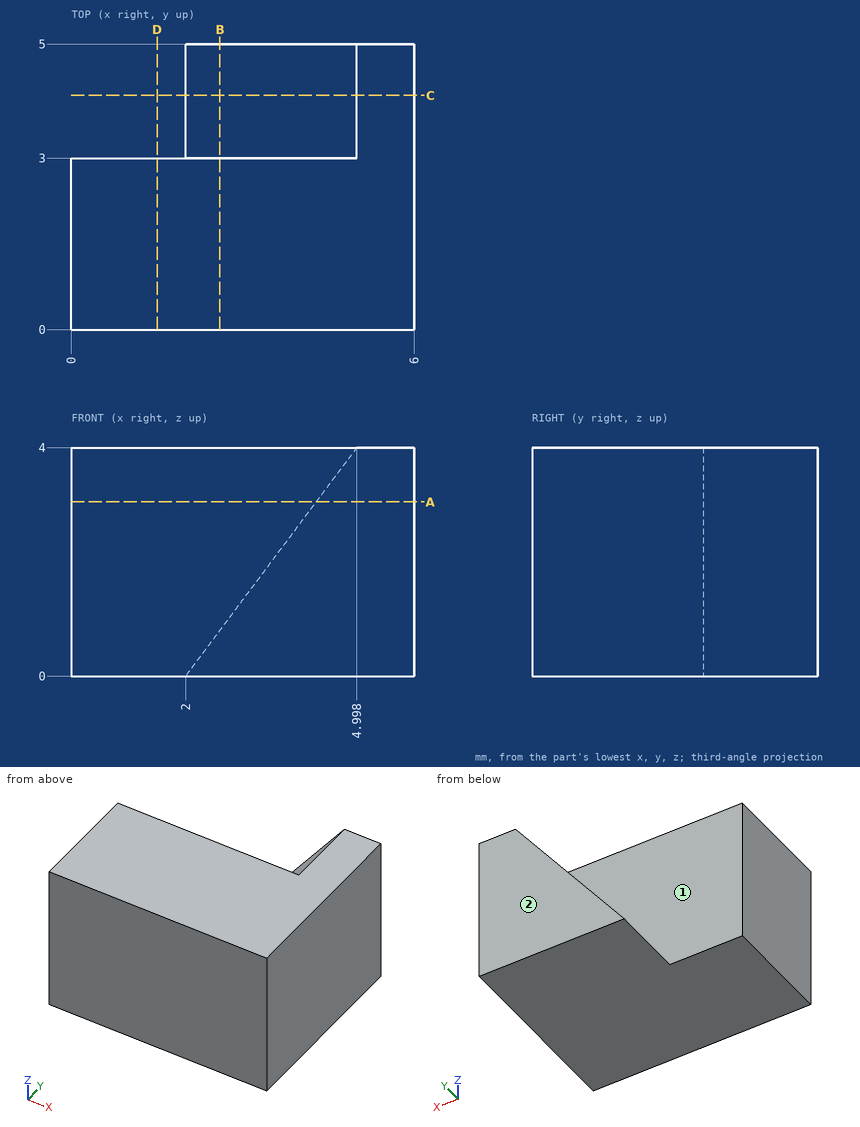
Part print with two shaded views. Sizes in mm from the minimum x, y, z corner. A direction names the side the tool comes from. Round coordinates to 2 decimals unless told otherwise and drop trailing zeros. Loops run counter-clockwise (first coordinate to the right, second up) from the corner with the lowest first, then second, coordinate; pieces in that order, holes last.
Item 1: Drill centre lines: line 1 along Y through (x, z) = (1.9, 1.45); line 2 along X through (y, z) = (4.45, 3.2); line 3 along X through (y, z) = (3.5, 1.85). Where is each one in solid material? Low to high.
Item 2: Which spindle directions (+Z, -Z, +X, -X, +Y, -Y) get a long thin tool onto all of the face, cutting with end or side? Do the marked faces 1 and 2. Say none if no direction does.
Item 3: Saw through at A-A (z = 3.05). List the corners of the cut face in (x, y), then the cut area to 3 significant figures.
Item 4: Saw through at D-D (x = 1.5). List the corners of the cut face in (y, z), then the cut area to 3 significant figures.
Item 5: Saw through at B-B (x = 2.6). List the corners of the cut face in (y, z), then the cut area to 3 significant figures.
Item 6: Saw through at C-C (y = 4.1). List the corners of the cut face in (x, z), then the cut area to 3 significant figures.
Worked answers:
1. line 1: y = 0 to 3
1. line 2: x = 4.4 to 6
1. line 3: x = 3.39 to 6
2. face 1: +Z, -X, +Y
2. face 2: +Z, -Z, +X, -X, +Y
3. outline: (0, 0) - (6, 0) - (6, 5) - (4.29, 5) - (4.29, 3) - (0, 3) - close
3. area: 21.4 mm2
4. outline: (0, 0) - (3, 0) - (3, 4) - (0, 4) - close
4. area: 12.0 mm2
5. outline: (0, 0) - (5, 0) - (5, 0.8) - (3, 0.8) - (3, 4) - (0, 4) - close
5. area: 13.6 mm2
6. outline: (2, 0) - (6, 0) - (6, 4) - (5, 4) - close
6. area: 10.0 mm2
